Work out the finished part from the listing and answer in its coordinate system (mm). Face numbers are marked on the shaded views. Give positions to 0.01 mm unless a question says otherwise; leave off trailing zeros. Order: outer loops, then holes, each group sorted by start corner. A loop starts at its lowest first (then second) coordinate and runs counter-clockwise, first axis right, second up.
```python
from build123d import *

# Parameters (mm, degrees)
BOSS_EXTRUDE1_DEPTH = 8.5
BOSS_EXTRUDE2_DEPTH = 2
BOSS_EXTRUDE3_DEPTH = 8.5


with BuildPart() as part:
    # Sketch1 → Boss-Extrude1 (new body)
    with BuildSketch(Plane(origin=(0, 0, 0), x_dir=(1, 0, 0), z_dir=(0, 1, 0))):
        with BuildLine():
            ThreePointArc((-18.5, 0), (0, 18.5), (18.5, 0))
            Line((18.5, 0), (20.5, 0))
            ThreePointArc((20.5, 0), (0, 20.5), (-20.5, 0))
            Line((-20.5, 0), (-18.5, 0))
        make_face()
    extrude(amount=BOSS_EXTRUDE1_DEPTH)

    # Sketch2 → Boss-Extrude2 (add)
    with BuildSketch(Plane(origin=(0, 8.5, 0), x_dir=(1, 0, 0), z_dir=(0, 1, 0))):
        with BuildLine():
            Line((-19.5, 0), (-20.5, 0))
            ThreePointArc((-20.5, 0), (0, 20.5), (20.5, 0))
            Line((20.5, 0), (19.5, 0))
            ThreePointArc((19.5, 0), (0, 19.5), (-19.5, 0))
        make_face()
    extrude(amount=BOSS_EXTRUDE2_DEPTH)

    # Sketch3 → Boss-Extrude3 (add)
    with BuildSketch(Plane(origin=(0, 10.5, 0), x_dir=(1, 0, 0), z_dir=(0, 1, 0))):
        with BuildLine():
            Line((-20.5, 0), (-18.5, 0))
            ThreePointArc((-18.5, 0), (0, 18.5), (18.5, 0))
            Line((18.5, 0), (20.5, 0))
            ThreePointArc((20.5, 0), (0, 20.5), (-20.5, 0))
        make_face()
    extrude(amount=BOSS_EXTRUDE3_DEPTH)


solid = part.part
```
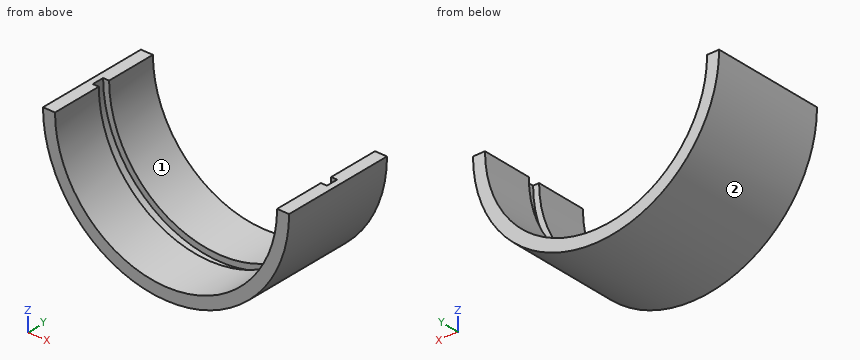
1. The mould has two halves that part along X. Classify the marked faces 1 and 2: pulls with the +X half, pulls with the -X half, needs draft (parallel to the pull), parting line crosses it, or undercut.
Findings below:
face 1: undercut
face 2: parting line crosses it
2. Straight lines are drawn through the part: probe 1 along X at (y, z) = (1.5, -13.75); probe 2 along X at (y, z) = (7.75, -6); probe 3 along Z at (x, y) = (8, 2). For each, find the intervals that lie inside material, in ascending order.
Findings below:
probe 1: x = -15.2 to -12.38, 12.38 to 15.2
probe 2: x = -19.6 to -17.5, 17.5 to 19.6
probe 3: z = -18.87 to -16.68
3. The part is cut by section D-D (y = 2.5). Write down the section's boundary in (x, z), then the cut area to 3 significant figures.
Findings below:
outline: (-20.5, 0) arc R20.5 ccw to (20.5, 0) - (18.5, 0) arc R18.5 cw to (-18.5, 0) - close
area: 123 mm2
4. The part is cut by section C-C (z = -19). Write down the section's boundary in (x, y), then the cut area to 3 significant figures.
Findings below:
outline: (-7.7, 0) - (7.7, 0) - (7.7, 19) - (-7.7, 19) - close; hole (-4.39, 8.5) - (4.39, 8.5) - (4.39, 10.5) - (-4.39, 10.5) - close
area: 275 mm2
5. The part is cut by section A-A (z = -10.5). Write down the section's boundary in (x, y).
Findings below:
outline: (-17.61, 0) - (-15.23, 0) - (-15.23, 8.5) - (-16.43, 8.5) - (-16.43, 10.5) - (-15.23, 10.5) - (-15.23, 19) - (-17.61, 19) - close; (15.23, 0) - (17.61, 0) - (17.61, 19) - (15.23, 19) - (15.23, 10.5) - (16.43, 10.5) - (16.43, 8.5) - (15.23, 8.5) - close
6. Given P1, Ø4, axis at x = 14.5, y = 13, coming from the -Z side; P2, Ø6, axis at y = 2, z = -3.5, coming from the -X side; P3, Ø2, axis at y = 11, z = -16, coming from the +X side, each flat-ended and moving along its own axis, determine where each tip first touches the part or whether it passes through.
Findings below:
P1: stops at z = -16.25
P2: stops at x = -20.49
P3: stops at x = 13.97
7. The part is cut by section B-B (x = 0). Write down the section's boundary in (y, z), then the cut area to 3 significant figures.
Findings below:
outline: (0, -20.5) - (19, -20.5) - (19, -18.5) - (10.5, -18.5) - (10.5, -19.5) - (8.5, -19.5) - (8.5, -18.5) - (0, -18.5) - close
area: 36.0 mm2
